Input: dimensioned drawing with shaded views. Units: mm. Origin: part minimum x, y, z. Coordinates: 2 decimals unless noted, no trailing zeros. Loops run counter-clockwise (first coordinate to the right, second up) from the corner with the lowest first, then second, coordinate; pieces in that order, holes last. Notation, with made-up numbers: (-6, 76) -> (32, 76) arc R15 ccw to (32, 94) -> close; hole circle Ø2 at (87, 35.25). An arc over 180 degrees is marked (long way). Answer as CSV lines item,"result".
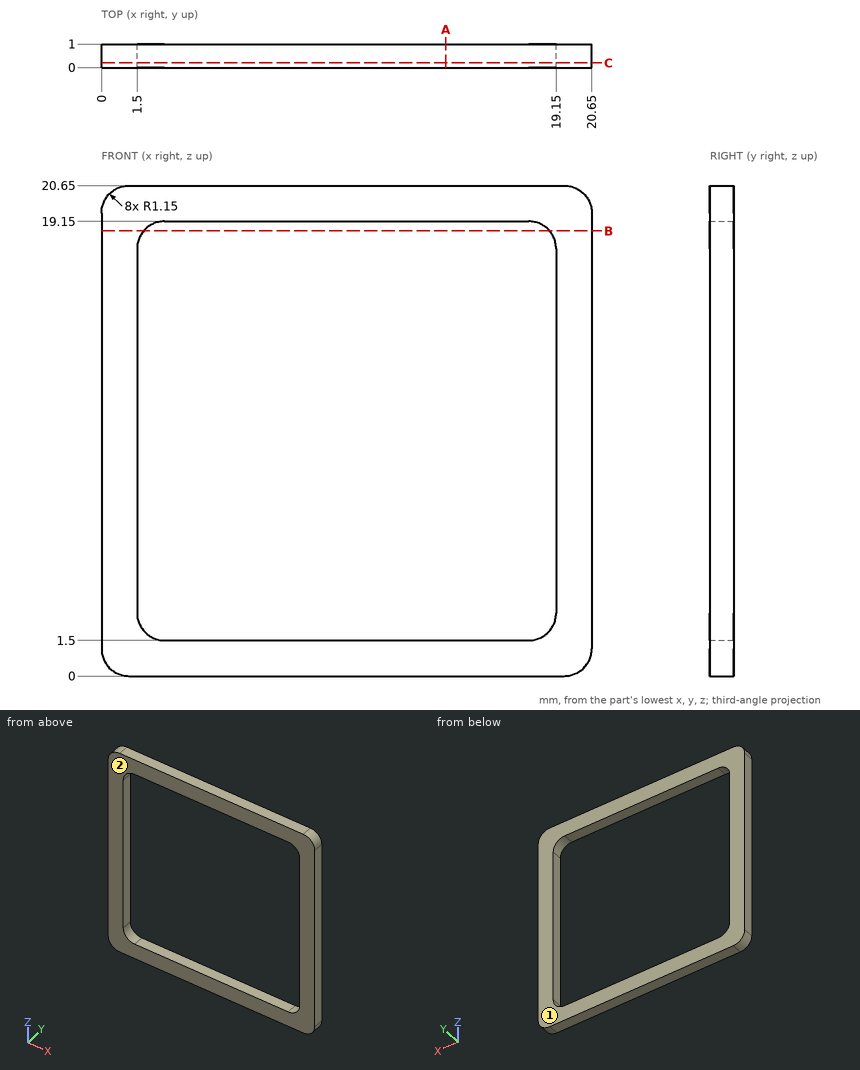
(1) Draft query along Y for the marked faces 1 and 2. Return one class per face: released by +Y, released by -Y, zero draft, split by the parting line, or undercut.
Computed values:
face 1,"released by +Y"
face 2,"released by -Y"
(2) Cut plane B-B (z = 18.75). Return the cut outline in (x, y).
Computed values:
outline,"(0, 0) -> (1.78, 0) -> (1.78, 1) -> (0, 1) -> close; (18.87, 0) -> (20.65, 0) -> (20.65, 1) -> (18.87, 1) -> close"
(3) Cut plane A-A (x = 14.5). Return the cut outline in (y, z).
Computed values:
outline,"(0, 0) -> (1, 0) -> (1, 1.5) -> (0, 1.5) -> close; (0, 19.15) -> (1, 19.15) -> (1, 20.65) -> (0, 20.65) -> close"
(4) Material intervals for L1, parallel to X at y = 0.7, z = 7.75; L2, parallel to Z at x = 19, y = 0.95, sorted ascending. Write a range as [from, to].
Computed values:
L1,"[0, 1.5], [19.15, 20.65]"
L2,"[0, 2.08], [18.57, 20.65]"
(5) Cut plane C-C (y = 0.2). Return the cut outline in (x, z).
Computed values:
outline,"(0, 1.15) arc R1.15 ccw to (1.15, 0) -> (19.5, 0) arc R1.15 ccw to (20.65, 1.15) -> (20.65, 19.5) arc R1.15 ccw to (19.5, 20.65) -> (1.15, 20.65) arc R1.15 ccw to (0, 19.5) -> close; hole (1.5, 2.65) arc R1.15 ccw to (2.65, 1.5) -> (18, 1.5) arc R1.15 ccw to (19.15, 2.65) -> (19.15, 18) arc R1.15 ccw to (18, 19.15) -> (2.65, 19.15) arc R1.15 ccw to (1.5, 18) -> close"
